Answer from the drawing. Dimensions are ordinates in mm from the lowest x, y and z of the part. Coordinates: 2 decimals unless noted, no trailing zeros. Order: outer loops, then holes, each group sorted by start corner. A loop starts at its lowest first (then second) coordinate and runs counter-clockwise, first axis right, second up. Notation, with made-up numbers: (21.25, 50) -> (54.25, 50) arc R26 cw to (54.25, 76) -> close; hole circle Ø3 at (-15, 85). An arc over 180 degrees is marked (long way). Answer in a Markdown table with one row per item.
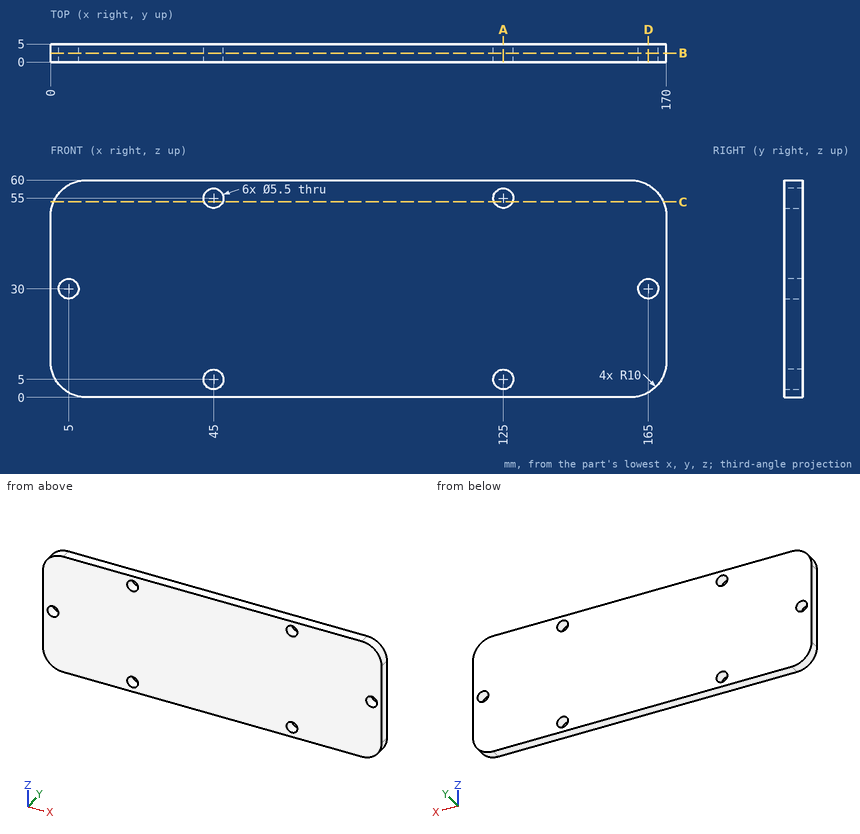
Q1. The part is cut by section D-D (x = 165). Write down the section's boundary in (y, z), then the cut area to 3 significant figures.
Outcome:
| item | result |
|---|---|
| outline | (0, 1.34) -> (5, 1.34) -> (5, 27.25) -> (0, 27.25) -> close; (0, 32.75) -> (5, 32.75) -> (5, 58.66) -> (0, 58.66) -> close |
| area | 259 mm² |
Q2. The part is cut by section B-B (y = 2.45). Write down the section's boundary in (x, z).
Outcome:
| item | result |
|---|---|
| outline | (0, 10) arc R10 ccw to (10, 0) -> (160, 0) arc R10 ccw to (170, 10) -> (170, 50) arc R10 ccw to (160, 60) -> (10, 60) arc R10 ccw to (0, 50) -> close; hole circle Ø5.5 at (5, 30); hole circle Ø5.5 at (45, 5); hole circle Ø5.5 at (45, 55); hole circle Ø5.5 at (125, 5); hole circle Ø5.5 at (125, 55); hole circle Ø5.5 at (165, 30) |
Q3. Consider line 1 (X direction, y = 1.7, z = 55); line 2 (Z direction, x = 42.5, y = 2.7); line 3 (Z direction, x = 44, y = 2.25). Determine where each line is inside the solid, lowest interval first.
Outcome:
| item | result |
|---|---|
| line 1 | 1.34 to 42.25, 47.75 to 122.25, 127.75 to 168.66 |
| line 2 | 0 to 3.85, 6.15 to 53.85, 56.15 to 60 |
| line 3 | 0 to 2.44, 7.56 to 52.44, 57.56 to 60 |
Q4. The part is cut by section C-C (z = 54). Write down the section's boundary in (x, y).
Outcome:
| item | result |
|---|---|
| outline | (0.83, 0) -> (42.44, 0) -> (42.44, 5) -> (0.83, 5) -> close; (47.56, 0) -> (122.44, 0) -> (122.44, 5) -> (47.56, 5) -> close; (127.56, 0) -> (169.17, 0) -> (169.17, 5) -> (127.56, 5) -> close |
Q5. The part is cut by section A-A (x = 125). Write down the section's boundary in (y, z), then the cut area to 3 significant figures.
Outcome:
| item | result |
|---|---|
| outline | (0, 0) -> (5, 0) -> (5, 2.25) -> (0, 2.25) -> close; (0, 7.75) -> (5, 7.75) -> (5, 52.25) -> (0, 52.25) -> close; (0, 57.75) -> (5, 57.75) -> (5, 60) -> (0, 60) -> close |
| area | 245 mm² |
